from build123d import *

# Parameters (mm, degrees)
F0_W      = 38.1
F0_H      = 38.1
F1_DEPTH  = 38.1
F6_DEPTH  = 50.8
F8_DEPTH  = 38.1
F9_W      = 25.4
F9_H      = 7.62
F10_DEPTH = 38.1


with BuildPart() as f1:
    # F0 (on Front) → F1 (new body)
    with BuildSketch(Plane.XZ):
        with Locations((19.05, 19.05)):
            Rectangle(F0_W, F0_H)
    extrude(amount=F1_DEPTH)

    # F5 (on offset) → F6 (cut)
    with BuildSketch(Plane.YZ.offset(38.1)):
        Polygon((-11.43, 11.31845), (-6.35, 38.1), (-31.75, 38.1), (-26.67, 11.672141), (-21.59, 28.575), (-16.51, 28.575), align=None)
        Polygon((-31.75, 0), (-38.1, 38.1), (-38.1, 0), align=None)
        Polygon((-25.4, 0), (-12.7, 0), (-19.05, 15.875), align=None)
        Polygon((-6.35, 0), (0, 0), (0, 38.1), align=None)
    extrude(amount=-F6_DEPTH, mode=Mode.SUBTRACT)

    # F7 (on offset) → F8 (cut)
    with BuildSketch(Plane.XZ.offset(38.1)):
        Polygon((0, 38.1), (0, 0), (6.35, 38.1), align=None)
        Polygon((25.4, 38.1), (12.7, 38.1), (19.05, 22.225), align=None)
        Polygon((31.75, 38.1), (38.1, 0), (38.1, 38.1), align=None)
        Polygon((11.43, 22.225), (6.35, 0), (31.75, 0), (26.67, 22.225), (21.59, 9.525), (16.51, 9.525), align=None)
    extrude(amount=-F8_DEPTH, mode=Mode.SUBTRACT)

    # F9 (on offset) → F10 (cut)
    with BuildSketch(Plane.XY.offset(38.1)):
        with Locations((12.7, -26.67)):
            Rectangle(F9_W, F9_H)
        with Locations((25.4, -11.43)):
            Rectangle(F9_W, F9_H)
    extrude(amount=-F10_DEPTH, mode=Mode.SUBTRACT)


solid = f1.part
Geometry: final body of the model. Coordinates: model frame, mm. A direction names the side the tool comes from. Give positions to 0.01 mm unless a question says otherwise; leave off trailing zeros. Loops run counter-clockwise (first coordinate to the right, second up) from the corner with the lowest first, then second, coordinate; pieces in that order, holes last. Notation, with made-up numbers: M -4.5,26 L 0.5,26 A11 ccw 0.5,31 Z; hole C -4,-18.75 d7. An arc over 180 degrees is marked long. Put each result on its own line as item: value. Start each with the question number.
1) Cut plane B-B (z = 8.5). Output: boundary loops of the cut face in (x, y).
2) Cut plane D-D (z = 16.5). Give the number of separate pieces and of enclosed holes in the cut face, then the cut area to 3 significant figures.
3) Cut plane A-A (z = 33.5). Output: boundary loops of the cut face in (x, y).
4) Access query for faces 1 (the flat face through (19, -32, 9.525)), 2 (the flat face through (8.727, -8.926, 24.522)), 3 (the flat face through (25, -15.24, 19)), 4 (the flat face through (15.83, -3.86, 30.27)), 5 (the flat face through (5.06, -15.83, 7.83)). Directions: +Z, -Z, +X, -X, +Y, -Y. A direction counts if a zero-diameter tool reaches every point of the face in a straight line with its end or side. Return the directions, or none.
5) Pull-direction query (Y, two-part tool) for faces 6 (the flat face through (19.32, -3.13, 19.32)), 7 (the flat face through (28, -19, 28.575)), 8 (the flat face through (34.175, -4.71, 23.55)); classes: pulls with the +Y half, pulls with the -Y half, needs draft (parallel to the pull), parting line crosses it, or undercut.
6) Contact query for flat-ended pins moving along their axis: pin 1 (3 mm diameter, centred on y = -10, z = 16.5, fed in from +X); pin 2 (8 mm diameter, centred on y = -32.5, z = 33.5, fed in from +X); pin 3 (0.5 mm diameter, centred on y = -14, z = 22, fed in from +X); pin 4 (6 mm diameter, centred on x = 7, z = 19, fed in from -Y). Output: stop coordinate, or through.
7) Cut plane C-C (y = -34.5). Output: boundary loops of the cut face in (x, z) (3 decimals), then the cut area to 3 significant figures.
8) Ray query, line 1 along Y through (x, z) = (32.5, 15.5); line 2 along X through (y, z) = (-6, 10); line 3 along Y through (x, z) = (29, 25). Return the intervals inside material, ascending.
Verdict:
1. outline: M 1.42,-33.17 L 8.29,-33.17 L 8.29,-30.48 L 1.42,-30.48 Z; M 1.42,-22.86 L 8.29,-22.86 L 8.29,-22 L 1.42,-22 Z; M 1.42,-16.1 L 8.29,-16.1 L 8.29,-4.93 L 1.42,-4.93 Z; M 29.81,-33.17 L 36.68,-33.17 L 36.68,-22 L 29.81,-22 Z; M 29.81,-16.1 L 36.68,-16.1 L 36.68,-15.24 L 29.81,-15.24 Z; M 29.81,-7.62 L 36.68,-7.62 L 36.68,-4.93 L 29.81,-4.93 Z
2. separate pieces: 9
2. enclosed holes: 0
2. area: 474 mm2
3. outline: M 5.58,-37.33 L 14.54,-37.33 L 14.54,-30.87 L 5.58,-30.87 Z; M 5.58,-7.22 L 14.54,-7.22 L 14.54,-0.77 L 5.58,-0.77 Z; M 23.56,-37.33 L 32.52,-37.33 L 32.52,-30.87 L 23.56,-30.87 Z; M 23.56,-7.22 L 32.52,-7.22 L 32.52,-0.77 L 23.56,-0.77 Z
4. face 1: -Z, +Y, -Y
4. face 2: +Z, +X, -X
4. face 3: +Z, -Z, +X
4. face 4: +Z, +Y, -Y
4. face 5: -Z, +X, -X
5. face 6: pulls with the +Y half
5. face 7: undercut
5. face 8: needs draft
6. pin 1: x = 10.46
6. pin 2: x = 33.18
6. pin 3: through
6. pin 4: y = -35.42
7. outline: M 2.75,16.5 L 10.121,16.5 L 11.43,22.225 L 13.72,16.5 L 24.38,16.5 L 26.67,22.225 L 27.979,16.5 L 35.35,16.5 L 31.75,38.1 L 25.4,38.1 L 19.05,22.225 L 12.7,38.1 L 6.35,38.1 Z
7. area: 505 mm2
8. line 1: -34.33 to -27.41, -25.52 to -19.2, -18.9 to -15.24, -7.62 to -3.77
8. line 2: 1.67 to 8.64, 16.32 to 21.78, 29.46 to 36.43
8. line 3: -35.92 to -29.23, -22.66 to -15.46, -7.62 to -2.18
